```python
from build123d import *

# Parameters (mm, degrees)
F1_DEPTH  = 48.5
F2_R      = 4.5
F2_R_2    = 1.5
F3_DEPTH  = 6
F4_W      = 51
F4_H      = 78
F4_R      = 5
F5_DEPTH  = 5
F7_DEPTH  = 1
F9_DEPTH  = 1
F11_DEPTH = 97
F12_DEPTH = 97
F13_W     = 15
F13_H     = 50
F14_DEPTH = 30
F16_DEPTH = 2


with BuildPart() as f1:
    # F0 (on Front) → F1 (new body, symmetric)
    with BuildSketch(Plane.XZ):
        with BuildLine():
            Line((-80.49844719, 0), (0, 33))
            Line((0, 33), (16.4209198648, 33))
            Line((16.4209198648, 33), (16.4209198648, 11.8303052739))
            Line((16.4209198648, 11.8303052739), (18.6015999846, 11.8303052739))
            Line((18.6015999846, 11.8303052739), (18.6015999846, 26.4569012833))
            ThreePointArc((18.6015999846, 26.4569012833), (24.7826070747, 32.9963067716), (31.3933508991, 26.8916578155))
            ThreePointArc((31.3933508991, 26.8916578155), (31.4, 26.6), (31.3933508991, 26.3083421845))
            Line((31.3933508991, 26.3083421845), (31.3933508991, 11.8303052739))
            Line((31.3933508991, 11.8303052739), (33.3968422327, 11.8303052739))
            Line((33.3968422327, 11.8303052739), (33.3968422327, 26.3696947261))
            Line((33.3968422327, 26.3696947261), (33.3968422327, 26.8303052739))
            ThreePointArc((33.3968422327, 26.8303052739), (30.8577058521, 32.62057158), (25, 35))
            Line((25, 35), (-0.3940335036, 35))
            Line((-0.3940335036, 35), (-82.49844719, 1.3416407865))
            Line((-82.49844719, 1.3416407865), (-82.49844719, -15))
            Line((-82.49844719, -15), (-80.49844719, -15))
            Line((-80.49844719, -15), (-80.49844719, 0))
        make_face()
    extrude(amount=F1_DEPTH, both=True)

    # F2 (on face) → F3 (join)
    with BuildSketch(Plane(origin=(-11.5818217717, 0, 28.2520808561), x_dir=(0.9252695079, 0, 0.3793103448), z_dir=(0.3793103448, 0, -0.9252695079))):
        with Locations((17.1811336159, 44)):
            Circle(F2_R)
        with Locations((17.1811336159, 44)):
            Circle(F2_R_2, mode=Mode.SUBTRACT)
        with BuildLine():
            ThreePointArc((-43.3188663841, -44), (-51.0008468994, -40.8180194847), (-47.8188663841, -48.5))
            ThreePointArc((-47.8188663841, -48.5), (-44.6368858688, -47.1819805153), (-43.3188663841, -44))
        make_face()
        with Locations((-47.8188663841, -44)):
            Circle(F2_R_2, mode=Mode.SUBTRACT)
        with BuildLine():
            ThreePointArc((-47.8188663841, 48.5), (-51.0008468994, 40.8180194847), (-43.3188663841, 44))
            ThreePointArc((-43.3188663841, 44), (-44.6368858688, 47.1819805153), (-47.8188663841, 48.5))
        make_face()
        with Locations((-47.8188663841, 44)):
            Circle(F2_R_2, mode=Mode.SUBTRACT)
        with Locations((17.1811336159, -44)):
            Circle(F2_R)
        with Locations((17.1811336159, -44)):
            Circle(F2_R_2, mode=Mode.SUBTRACT)
    extrude(amount=F3_DEPTH)

    # F4 (on face) → F5 (cut)
    with BuildSketch(Plane(origin=(-12.3404424613, 0, 30.102619872), x_dir=(0.9252695079, 0, 0.3793103448), z_dir=(-0.3793103448, 0, 0.9252695079))):
        with Locations((-24.2887251171, 0.5)):
            Rectangle(F4_W, F4_H)
        with Locations((-67.3243994072, -36.5)):
            Circle(F4_R)
    extrude(amount=-F5_DEPTH, mode=Mode.SUBTRACT)

    # F6 (on face) → F7 (join)
    with BuildSketch(Plane.XZ.offset(48.5)):
        Polygon((-80.49844719, -15), (16.4209198648, 11.8303052739), (16.4209198648, 33), (5.040577039, 33), (0, 33), (-55.8271606545, 10.1138901941), (-80.49844719, 0), align=None)
    extrude(amount=-F7_DEPTH)

    # F8 (on face) → F9 (join)
    with BuildSketch(Plane(origin=(0, 48.5, 0), x_dir=(-1, 0, 0), z_dir=(0, 1, 0))):
        Polygon((-16.4209198648, 11.8303052739), (80.49844719, -15), (80.49844719, 0), (55.8271607407, 10.1138901587), (0, 33), (-5.040577039, 33), (-16.4209198648, 33), align=None)
    extrude(amount=-F9_DEPTH)

    # F10 (on face) → F11 (join)
    with BuildSketch(Plane(origin=(0, 48.5, 0), x_dir=(-1, 0, 0), z_dir=(0, 1, 0))):
        with BuildLine():
            Line((82.49844719, -13.8338189837), (82.49844719, -15))
            ThreePointArc((82.49844719, -15), (87.3045087217, -6.8291796068), (82.49844719, 1.3416407865))
            Line((82.49844719, 1.3416407865), (82.49844719, 0.1754597702))
            ThreePointArc((82.49844719, 0.1754597702), (86.3045087217, -6.8291796068), (82.49844719, -13.8338189837))
        make_face()
    extrude(amount=-F11_DEPTH)

    # F10 (on face) → F12 (join)
    with BuildSketch(Plane(origin=(0, 48.5, 0), x_dir=(-1, 0, 0), z_dir=(0, 1, 0))):
        with BuildLine():
            Line((82.49844719, 0.1754597702), (82.49844719, -13.8338189837))
            ThreePointArc((82.49844719, -13.8338189837), (86.3045087217, -6.8291796068), (82.49844719, 0.1754597702))
        make_face()
    extrude(amount=-F12_DEPTH)

    # F13 (on face) → F14 (cut)
    with BuildSketch(Plane.XY.offset(35)):
        with Locations((17.5, 0)):
            Rectangle(F13_W, F13_H)
        with Locations((32.5, 0)):
            Rectangle(F13_W, F13_H)
    extrude(amount=-F14_DEPTH, mode=Mode.SUBTRACT)

    # F15 (on face) → F16 (cut)
    with BuildSketch(Plane(origin=(0, 48.5, 0), x_dir=(-1, 0, 0), z_dir=(0, 1, 0))):
        Polygon((38.2937746964, 4.3324337855), (17.9378455219, 12.6772613717), (16.0412937978, 8.0509138321), (36.3972229723, -0.2939137541), align=None)
    extrude(amount=-F16_DEPTH, mode=Mode.SUBTRACT)


solid = f1.part
```
Here's how the part is built. I have some questions about the finished solid (model axes, mm). A direction names the side the tool comes from. Give positions to 0.01 mm unless a question says otherwise; leave off trailing zeros. Write each loop counter-clockwise with the first axis right and the second up, starting at its lowest first coordinate (ties: lowest second). Pieces come first, ordered by that corner, then holes. Notation, with made-up numbers: M -28,54 L 22,54 A36 cw 22,93 Z; hole C 66,85 d6. An arc over 180 degrees is marked long. Put each result on its own line as item: value. Start each with the question number.
Item 1: If we section it at C-C, the plane y = 37.5: Write out the boundary of the cut face in (x, z).
Item 2: If we section it at A-A, the plane y = 22: Write out the boundary of the cut face in (x, z).
Item 3: If we section it at B-B, the plane x = 22: Write out the boundary of the cut face in (y, z).
Item 4: Will these pins go through, and if not, where does the flat tip stop? pin 1 (5 mm diameter, centred on x = -67.5, y = -23.5, fed in from -Z); pin 2 (12 mm diameter, centred on x = 17.5, y = 30, fed in from -Z); pin 3 (12.5 mm diameter, centred on x = 13.5, y = 0.5, fed in from +Z).
Item 5: Thinking about a two-plate mould opening in X: for faces 6 (the flat face through (-59.117, -0.679, 10.927)), 7 (the flat face through (16.421, 36, 23)), 8 (the flat face through (33.397, 37, 19)), 9 (the flat face through (18, -25, 26)), which applies, +X half, -X half, draft (parallel to the pull), parting line (faces both ways), or undercut?
Item 6: On a 3-axis mill with a long thin cutter (end or side, diameter ignored), from which of +Z, -Z, +X, -X, +Y, -Y can I reach the whole of each face in a straight line? I mean faces 1 (the flat face through (31.393, -37, 19)), 2 (the flat face through (-52.68, 42.56, 4.92)), 3 (the flat face through (-28.258, 48.007, 8.446)), 4 (the flat face through (18, 25, 27)), 5 (the flat face through (-55.847, -44.021, 10.106)). Say none if no direction works.
Item 7: I need wall thicknesses on L1, parallel to X at y = -41, z = 19; L2, parallel to Y at x = -9.5, z = 19; L3, parallel to X at y = 29, z = 24. Which ranges of each line are inside material? Lowest first, please. Write a range as from..to.
Values:
1. outline: M -82.5,-15 L -80.5,-15 L -80.5,0 L -57.65,9.37 L -58.41,11.22 L -82.5,1.34 A9.35 ccw Z; M -11.22,30.56 L -10.46,28.71 L 0,33 L 16.42,33 L 16.42,11.83 L 18.6,11.83 L 18.6,26.46 A6.4 cw long 31.39,26.31 L 31.39,11.83 L 33.4,11.83 L 33.4,26.83 A8.4 ccw 25,35 L -0.39,35 Z
2. outline: M -82.5,-15 L -80.5,-15 L -80.5,0 L -57.65,9.37 L -58.41,11.22 L -82.5,1.34 A9.35 ccw Z; M -11.22,30.56 L -10.46,28.71 L 0,33 L 10,33 L 10,35 L -0.39,35 Z
3. outline: M -48.5,32.25 L -25,32.25 L -25,35 L -48.5,35 Z; M 25,32.25 L 48.5,32.25 L 48.5,35 L 25,35 Z
4. pin 1: z = 4.3
4. pin 2: z = 11.83
4. pin 3: z = 35
5. face 6: -X half
5. face 7: undercut
5. face 8: +X half
5. face 9: draft
6. face 1: -Z, +Y, -Y
6. face 2: -Z, +X
6. face 3: +Y
6. face 4: +Z, -Z, +X
6. face 5: none
7. L1: -39.42..-34.15, 16.42..18.6, 31.39..33.4
7. L2: -48.5..-47.5, 47.5..48.5
7. L3: 16.42..18.6, 31.39..33.4
